Autodesk Inventor part; units mm, degrees
ref_plane "Work Plane1" through (-42, 0, 0) normal (1, 0, 0) x (0, 1, 0)
ref_plane "Work Plane2" through (-25, 0, 0) normal (1, 0, 0) x (0, 1, 0)
ref_plane "XZ Plane" through (0, 0, 0) normal (0, 1, 0) x (-1, 0, 0)
sketch "Sketch1" plane through (0, 0, 0) normal (0, 0, 1) x (1, 0, 0)
  circle A0 centre (0, 0) radius 5
  dimension "d0" = 10
extrude "Extrusion1" add sketch "Sketch1" against normal blind 50
ref_plane "Work Plane1" through (-42, 0, 0) normal (1, 0, 0) x (0, 1, 0)
sketch "Sketch2" plane through (-42, 0, 0) normal (1, 0, 0) x (0, 1, 0)
  line L0 (5, -50) -> (-5, -50)
  line L1 (-5, 0) -> (5, 0)
  line L2 (0, -60) -> (0, 10)
  line L3 (-2, 0) -> (2, 0)
  line L4 (2, 0) -> (2, -50)
  line L5 (2, -50) -> (-2, -50)
  line L6 (-2, -50) -> (-2, 0)
  dimension "d4" = 4
  dimension "d5" = 2
extrude "Extrusion2" add sketch "Sketch2" along normal blind 42
sketch "Sketch3" plane through (0, 0, 0) normal (0, 0, 1) x (1, 0, 0)
  arc A0 (-4.5826, -2) -> (-4.5826, 2) centre (0, 0) ccw
hole "Hole1" at (0, 0, 0) direction (0, 0, -1) diameter 6 end through all
ref_plane "Work Plane2" through (-25, 0, 0) normal (1, 0, 0) x (0, 1, 0)
sketch "Sketch4" plane through (-42, -2, -50) normal (0, -1, 0) x (1, 0, 0)
  line L0 (0, 0) -> (37.4174, 0)
  line L1 (17, 60) -> (17, -10)
  point P0 (17, 40)
  point P1 (17, 10)
  dimension "d16" = 30
  dimension "d17" = 10
hole "Hole2" at (-25, -2, -10) at (-25, -2, -40) direction (0, 1, 0) diameter 6.4 end through all countersink diameter 12.6 countersink angle 90
sketch "Sketch5" plane through (0, 0, -50) normal (0, 0, -1) x (-1, 0, 0)
  line L0 (42, -2) -> (4.5826, -2)
  line L1 (25, -7) -> (25, 7)
  line L2 (24.9, -2) -> (25, -1.9)
  line L3 (25, -1.9) -> (25.1, -2)
  dimension "d25" = 90
  dimension "d26" = 45
  dimension "d27" = 0.1
extrude "Extrusion3" cut sketch "Sketch5" against normal through all
fillet "Fillet1" radius 2 1 edges at (-42, -2, -25)
equation "\"d5\" = 0.5 * d4"
equation "\"d26\" = 0.5 * d25"
properties part number "23-225Z1" material "Aluminum-6061"
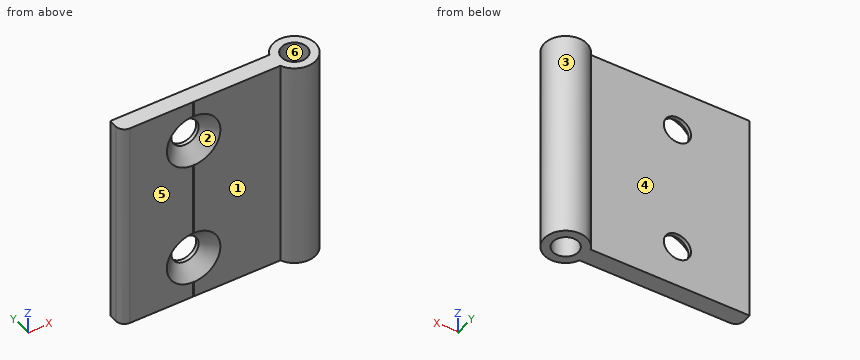
Could you check a few things on this model? Use its own coordinates, in mm. Face numbers are marked on the shaded views. A direction names the side the tool comes from. Give positions to 0.01 mm unless a question says otherwise; leave off trailing zeros. Loops run counter-clockwise (first coordinate to the right, second up) from the corner with the lowest first, then second, coordinate; pieces in that order, holes last. Notation, with made-up numbers: (9, 35) -> (61, 35) arc R24 ccw to (61, 57) -> close; hole circle Ø7 at (60.25, 2.25). An arc over 180 degrees is marked (long way). Return JSON: item names as keys, results as strings.
Item 1: If we section it at A-A on z = -40: List the corners of the cut face in (x, y) for me.
Geometry results:
{"outline": "(-42, 0) arc R2 ccw to (-40, -2) -> (-31.3, -2) -> (-28.2, 1.1) -> (-28.2, 2) -> (-42, 2) -> close; (-21.8, 1.1) -> (-18.7, -2) -> (-4.58, -2) arc R5 ccw (long way) to (-4.58, 2) -> (-21.8, 2) -> close; hole circle Ø6 at (0, 0)"}
Item 2: I'm going to push flat-ended pins straight in: pin 1 (4 mm diameter, centred on x = -25, z = -10, fed in from -Y); pin 2 (1.5 mm diameter, centred on y = 1.5, z = -16, fed in from +X); pin 3 (7.5 mm diameter, centred on x = -31, z = -35, fed in from -Y); pin 4 (3 mm diameter, centred on x = -21, z = -20, fed in from +Y). Where does each tip first touch, or does it pass through?
Geometry results:
{"pin 1": "passes through", "pin 2": "stops at x = 4.94", "pin 3": "stops at y = -2", "pin 4": "stops at y = 2"}
Item 3: If we section it at D-D on y = 4.25: List the corners of the cut face in (x, z) for me.
Geometry results:
{"outline": "(-2.63, -50) -> (2.63, -50) -> (2.63, 0) -> (-2.63, 0) -> close"}
Item 4: If we section it at C-C on z = -27: List the corners of the cut face in (x, y) for me, plus the area to 3 significant figures.
Geometry results:
{"outline": "(-42, 0) arc R2 ccw to (-40, -2) -> (-25.1, -2) -> (-25, -1.9) -> (-24.9, -2) -> (-4.58, -2) arc R5 ccw (long way) to (-4.58, 2) -> (-42, 2) -> close; hole circle Ø6 at (0, 0)", "area": "198 mm²"}
Item 5: If we section it at B-B on x = 0: List the corners of the cut face in (y, z) for me.
Geometry results:
{"outline": "(-5, -50) -> (-3, -50) -> (-3, 0) -> (-5, 0) -> close; (3, -50) -> (5, -50) -> (5, 0) -> (3, 0) -> close"}
Item 6: We'd pull the mould along Y, two halves only. Please class the marked faces 3, 4, 5 and 6: +Y half, -Y half, draft (parallel to the pull), parting line (faces both ways), or undercut.
Geometry results:
{"face 3": "parting line", "face 4": "+Y half", "face 5": "-Y half", "face 6": "undercut"}
Item 7: I need wall thicknesses on L1, parallel to Z at x = -25, y = 1.6; L2, parallel to Z at x = -27, y = 0.75; L3, parallel to X at y = 1.35, z = -40. Which ranges of each line are inside material? Lowest first, please. Write a range as from..to.
Geometry results:
{"L1": "z = -50..-43.2, -36.8..-13.2, -6.8..0", "L2": "z = -50..-42.93, -37.07..-12.93, -7.07..0", "L3": "x = -42..-28.2, -21.8..-2.68, 2.68..4.81"}
Item 8: Which directions (+Z, -Z, +X, -X, +Y, -Y) give clear straight access to the entire face, cutting with the end or side of a thin tool? Please do the marked faces 1 and 2.
Geometry results:
{"face 1": "+Z, -Z, -X, -Y", "face 2": "-Y"}
